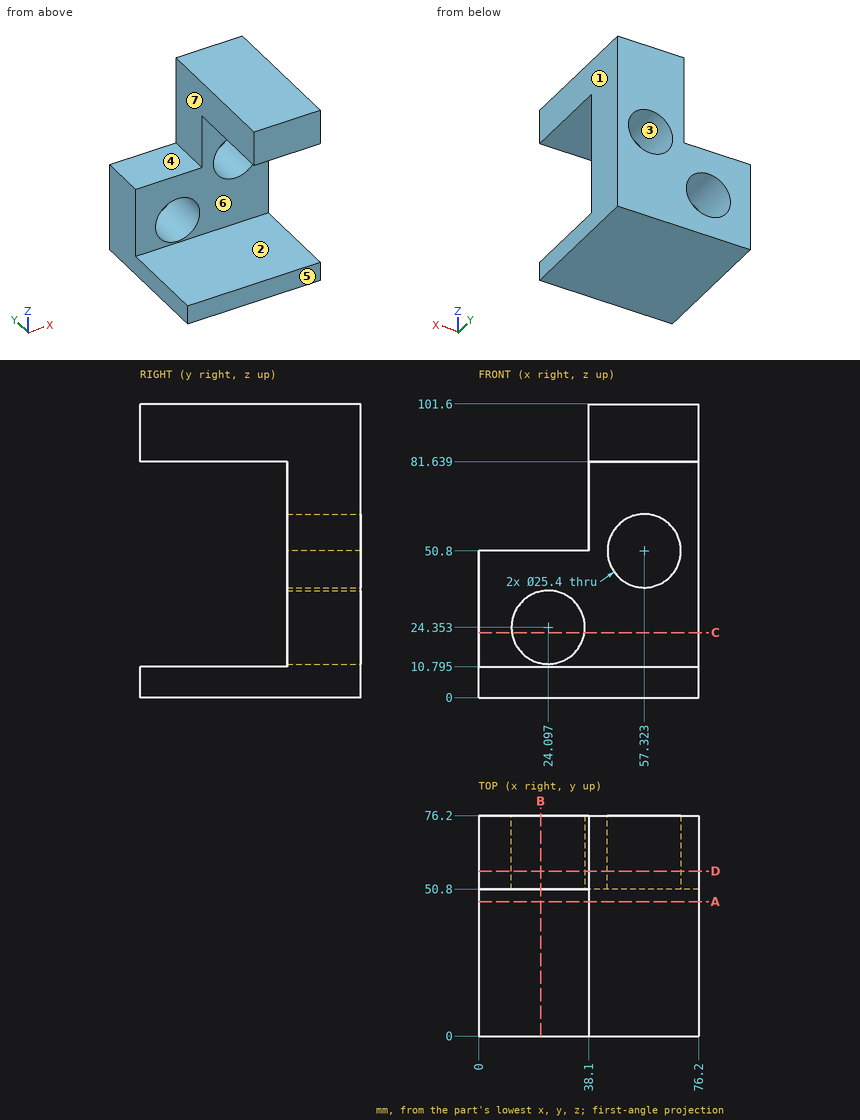
Input: dimensioned drawing with shaded views. Units: mm. Origin: part minimum x, y, z. A direction names the side the tool comes from. Round coordinates to 2 decimals unless told otherwise and drop trailing zeros. Order: outer loops, then holes, each group sorted by start corner. A loop starts at its lowest first (then second) coordinate and runs counter-clockwise, first axis right, second up. Notation, with made-up numbers: (45, 54) - (103, 54) arc R18 ccw to (103, 79) - close; hole circle Ø6 at (44.5, -7.5). An arc over 180 degrees is marked (long way). Use CSV: the item, a comma, the result in double quotes. Start each with the question number.
Q1. Mould query, pull axis Z, two halves, no side actions, for the marked faces 1, 2, 3 and 4. Classes: +Z half, -Z half, draft (parallel to the pull), parting line (faces both ways), or undercut.
Q2. Section query B-B (x = 21.5). Return loops of the section in (y, z) (1 decimal).
Q3. Access query for the marked faces 5, 6 and 7. Directions: +Z, -Z, +X, -X, +Y, -Y. A direction counts if a zero-diameter tool reaches every point of the face in a straight line with its end or side. Return the directions, or none.
Q4. Section query C-C (z = 22.5). Return loops of the section in (x, y), and give its area (3 significant figures).
Q5. Section query A-A (y = 46.5). Return loops of the section in (x, z) (1 decimal).
Q6. Material intervals for line 1 along Z through (x, y) = (55.5, 17) (1 decimal); line 2 along Y through (x, z) = (27, 50.5); line 3 along Z through (x, y) = (33, 50) (1 decimal), sorted ascending. Write a range as from..to.
Q7. First-contact query: pin 1 (12.5 mm diameter, centred on x = 26, y = 68, fed in from +Z); pin 2 (15 mm diameter, centred on y = 24, z = 85, fed in from -X). Flat tips, straight axial feed; report the tip coordinate or a pass-through.
Q8. Section query D-D (y = 57). Return loops of the section in (x, z).
Result set:
1,face 1,"draft"
1,face 2,"undercut"
1,face 3,"undercut"
1,face 4,"+Z half"
2,outline,"(0, 0) - (76.2, 0) - (76.2, 11.9) - (50.8, 11.9) - (50.8, 10.8) - (0, 10.8) - close; (50.8, 36.8) - (76.2, 36.8) - (76.2, 50.8) - (50.8, 50.8) - close"
3,face 5,"+Z, -Z, +X, -X, -Y"
3,face 6,"+X, -X, -Y"
3,face 7,"+Z, -X, +Y, -Y"
4,outline,"(0, 50.8) - (11.53, 50.8) - (11.53, 76.2) - (0, 76.2) - close; (36.66, 50.8) - (76.2, 50.8) - (76.2, 76.2) - (36.66, 76.2) - close"
4,area,"1,300 mm2"
5,outline,"(0, 0) - (76.2, 0) - (76.2, 10.8) - (0, 10.8) - close; (38.1, 81.6) - (76.2, 81.6) - (76.2, 101.6) - (38.1, 101.6) - close"
6,line 1,"z = 0..10.8, 81.6..101.6"
6,line 2,"y = 50.8..76.2"
6,line 3,"z = 0..10.8"
7,pin 1,"stops at z = 50.8"
7,pin 2,"stops at x = 38.1"
8,outline,"(0, 0) - (76.2, 0) - (76.2, 101.6) - (38.1, 101.6) - (38.1, 50.8) - (0, 50.8) - close; hole circle Ø25.4 at (24.1, 24.35); hole circle Ø25.4 at (57.32, 50.8)"
